```python
from build123d import *

# Parameters (mm, degrees)
SKETCH_1_W                = 130
SKETCH_1_H                = 15
EXTRUDE_1_DEPTH           = 8
CUT_EXTRUDE_10_REACH      = 133.107
SKETCH_17_R               = 3
CUT_EXTRUDE_12_REACH      = 133.107
SKETCH_15_R               = 3
SKETCH_22_W               = 8
SKETCH_22_H               = 8
EXTRUDE_7_DEPTH           = 5
CUT_EXTRUDE_18_DEPTH      = 1.5
SKETCH_25_W               = 4.62
SKETCH_25_H               = 1.5
CUT_EXTRUDE_19_DEPTH      = 4
FILLET_8_R                = 3
FILLET_9_R                = 2
FILLET_10_R               = 2
FILLET_11_R               = 3
CUT_EXTRUDE_20_DEPTH      = 15.5
CUT_EXTRUDE_20_DEPTH_BACK = 28.5
SKETCH_21_R               = 1
FILLET_12_R               = 10
FILLET_13_R               = 5


# Some blends are built 0.0001 mm under size
with BuildPart() as part:
    # 草图1 → 凸台-拉伸1 (new body)
    with BuildSketch(Plane(origin=(0, 0, 0), x_dir=(0, 0, -1), z_dir=(1, 0, 0))):
        with Locations((65, 7.5)):
            Rectangle(SKETCH_1_W, SKETCH_1_H)
    extrude(amount=EXTRUDE_1_DEPTH)

    # 草图17 → 切除-拉伸10 (cut, up to next)
    with BuildSketch(Plane.ZY, mode=Mode.PRIVATE) as cut_extrude_10_sk1:
        with Locations((-115, 7.5)):
            Circle(SKETCH_17_R)
    cut_extrude_10_tool1 = extrude(cut_extrude_10_sk1.sketch, amount=-CUT_EXTRUDE_10_REACH, mode=Mode.PRIVATE) & part.part
    # 草图17 → 切除-拉伸10 (cut, up to next)
    with BuildSketch(Plane.ZY, mode=Mode.PRIVATE) as cut_extrude_10_sk2:
        with Locations((-95, 7.5)):
            Circle(SKETCH_17_R)
    cut_extrude_10_tool2 = extrude(cut_extrude_10_sk2.sketch, amount=-CUT_EXTRUDE_10_REACH, mode=Mode.PRIVATE) & part.part
    # 草图17 → 切除-拉伸10 (cut, up to next)
    with BuildSketch(Plane.ZY, mode=Mode.PRIVATE) as cut_extrude_10_sk3:
        with Locations((-75, 7.5)):
            Circle(SKETCH_17_R)
    cut_extrude_10_tool3 = extrude(cut_extrude_10_sk3.sketch, amount=-CUT_EXTRUDE_10_REACH, mode=Mode.PRIVATE) & part.part
    # 草图17 → 切除-拉伸10 (cut, up to next)
    with BuildSketch(Plane.ZY, mode=Mode.PRIVATE) as cut_extrude_10_sk4:
        with Locations((-55, 7.5)):
            Circle(SKETCH_17_R)
    cut_extrude_10_tool4 = extrude(cut_extrude_10_sk4.sketch, amount=-CUT_EXTRUDE_10_REACH, mode=Mode.PRIVATE) & part.part
    # 草图17 → 切除-拉伸10 (cut, up to next)
    with BuildSketch(Plane.ZY, mode=Mode.PRIVATE) as cut_extrude_10_sk5:
        with Locations((-35, 7.5)):
            Circle(SKETCH_17_R)
    cut_extrude_10_tool5 = extrude(cut_extrude_10_sk5.sketch, amount=-CUT_EXTRUDE_10_REACH, mode=Mode.PRIVATE) & part.part
    add(cut_extrude_10_tool1.solids().sort_by_distance((0, 7.5, -115))[0], mode=Mode.SUBTRACT)
    add(cut_extrude_10_tool2.solids().sort_by_distance((0, 7.5, -95))[0], mode=Mode.SUBTRACT)
    add(cut_extrude_10_tool3.solids().sort_by_distance((0, 7.5, -75))[0], mode=Mode.SUBTRACT)
    add(cut_extrude_10_tool4.solids().sort_by_distance((0, 7.5, -55))[0], mode=Mode.SUBTRACT)
    add(cut_extrude_10_tool5.solids().sort_by_distance((0, 7.5, -35))[0], mode=Mode.SUBTRACT)

    # 草图15 → 切除-拉伸12 (cut, up to next)
    with BuildSketch(Plane.ZY, mode=Mode.PRIVATE) as cut_extrude_12_sk1:
        with Locations((-6.4, 7.5)):
            Circle(SKETCH_15_R)
    cut_extrude_12_tool1 = extrude(cut_extrude_12_sk1.sketch, amount=-CUT_EXTRUDE_12_REACH, mode=Mode.PRIVATE) & part.part
    add(cut_extrude_12_tool1.solids().sort_by_distance((0, 7.5, -6.4))[0], mode=Mode.SUBTRACT)

    # 草图22 → 凸台-拉伸7 (add)
    with BuildSketch(Plane(origin=(0, 15, 0), x_dir=(1, 0, 0), z_dir=(0, 1, 0))):
        with Locations((4, 6.4)):
            Rectangle(SKETCH_22_W, SKETCH_22_H)
    extrude_7 = extrude(amount=EXTRUDE_7_DEPTH)

    # 草图24 → 切除-拉伸18 (cut)
    with BuildSketch(Plane(origin=(0, 15, 0), x_dir=(1, 0, 0), z_dir=(0, 1, 0))):
        Polygon((4, 4.090598923), (6, 5.245299462), (6, 7.554700538), (4, 8.709401077), (2, 7.554700538), (2, 5.245299462), align=None)
    cut_extrude_18 = extrude(amount=CUT_EXTRUDE_18_DEPTH, mode=Mode.SUBTRACT)

    # 草图25 → 切除-拉伸19 (cut)
    with BuildSketch(Plane(origin=(8, 0, 0), x_dir=(0, 0, -1), z_dir=(1, 0, 0))):
        with Locations((6.4, 15.75)):
            Rectangle(SKETCH_25_W, SKETCH_25_H)
    cut_extrude_19 = extrude(amount=-CUT_EXTRUDE_19_DEPTH, mode=Mode.SUBTRACT)

    # 圆角8
    # the kernel refuses this fillet: 3 mm, written as the material it adds along each edge
    with BuildSketch(Plane(origin=(8, 15, -2.4), x_dir=(0, 1.5846583304811187e-12, 1.0), z_dir=(-1, 0, 0))) as fillet_8_piece_1:
        with BuildLine():
            CenterArc((3, 2.939387691), FILLET_8_R, 180, 78.463040967)
            Line((0, 2.939387691), (-0.06, 2.939387691))
            Line((-0.06, 2.939387691), (-0.06, 0))
            Line((-0.06, 0), (0, -0.06))
            ThreePointArc((0, -0.06), (1.2, -0.06), (2.388, -0.058787754))
            Line((2.388, -0.058787754), (2.4, 0))
        make_face()
    extrude(amount=8)
    with BuildSketch(Plane(origin=(0, 15, -10.4), x_dir=(0, 0, -1), z_dir=(1, 0, 0))) as fillet_8_piece_2:
        with BuildLine():
            CenterArc((FILLET_8_R, FILLET_8_R), FILLET_8_R, 180, 90)
            Line((0, FILLET_8_R), (-FILLET_8_R * 0.02, FILLET_8_R))
            Line((-FILLET_8_R * 0.02, FILLET_8_R), (-FILLET_8_R * 0.02, -FILLET_8_R * 0.02))
            Line((-FILLET_8_R * 0.02, -FILLET_8_R * 0.02), (FILLET_8_R, -FILLET_8_R * 0.02))
            Line((FILLET_8_R, -FILLET_8_R * 0.02), (FILLET_8_R, 0))
        make_face()
    extrude(amount=8)

    # 圆角9
    fillet_9_edges = [part.edges().sort_by_distance(p)[0] for p in [
        (4, 20, -2.4),
        (4, 20, -10.4),
    ]]
    fillet(fillet_9_edges, radius=FILLET_9_R - 0.0001)  # a hair under: the kernel refuses the full size

    # 镜向6: 凸台-拉伸7, 切除-拉伸18, 切除-拉伸19 across plane
    add(extrude_7.mirror(Plane.ZX.offset(7.5)))
    add(cut_extrude_18.mirror(Plane.ZX.offset(7.5)), mode=Mode.SUBTRACT)
    add(cut_extrude_19.mirror(Plane.ZX.offset(7.5)), mode=Mode.SUBTRACT)

    # 圆角10
    fillet_10_edges = [part.edges().sort_by_distance(p)[0] for p in [
        (4, -5, -10.4),
        (4, -5, -2.4),
    ]]
    fillet(fillet_10_edges, radius=FILLET_10_R)

    # 圆角11
    # the kernel refuses this fillet: 3 mm, written as the material it adds along each edge
    with BuildSketch(Plane(origin=(8, 0, -2.4), x_dir=(0, -1, 0), z_dir=(-1, 0, 0))) as fillet_11_piece_1:
        with BuildLine():
            CenterArc((2.939387691, 3), FILLET_11_R, 191.536959033, 78.463040967)
            Line((0, 2.4), (-0.058787754, 2.388))
            ThreePointArc((-0.058787754, 2.388), (-0.06, 1.2), (-0.06, 0))
            Line((-0.06, 0), (0, -0.06))
            Line((0, -0.06), (2.939387691, -0.06))
            Line((2.939387691, -0.06), (2.939387691, 0))
        make_face()
    extrude(amount=8)
    with BuildSketch(Plane(origin=(0, 0, -10.4), x_dir=(0, -1, 0), z_dir=(1, 0, 0))) as fillet_11_piece_2:
        with BuildLine():
            CenterArc((FILLET_11_R, FILLET_11_R), FILLET_11_R, 180, 90)
            Line((0, FILLET_11_R), (-FILLET_11_R * 0.02, FILLET_11_R))
            Line((-FILLET_11_R * 0.02, FILLET_11_R), (-FILLET_11_R * 0.02, -FILLET_11_R * 0.02))
            Line((-FILLET_11_R * 0.02, -FILLET_11_R * 0.02), (FILLET_11_R, -FILLET_11_R * 0.02))
            Line((FILLET_11_R, -FILLET_11_R * 0.02), (FILLET_11_R, 0))
        make_face()
    extrude(amount=8)

    # 草图21 → 切除-拉伸20 (cut, two sides: drawn at the far end of the back side and taken through both)
    with BuildSketch(Plane(origin=(0, 15, 0), x_dir=(1, 0, 0), z_dir=(0, 1, 0)).offset(-CUT_EXTRUDE_20_DEPTH_BACK)):
        with Locations(Location((4, 6.4, 0), (0, 0, 90))):
            Circle(SKETCH_21_R)
    extrude(amount=CUT_EXTRUDE_20_DEPTH + CUT_EXTRUDE_20_DEPTH_BACK, mode=Mode.SUBTRACT)

    # 圆角12
    fillet_12_edges = [part.edges().sort_by_distance(p)[0] for p in [
        (4, 15, 0),
        (4, 0, 0),
    ]]
    fillet(fillet_12_edges, radius=FILLET_12_R)

    # 圆角13
    fillet_13_edges = [part.edges().sort_by_distance(p)[0] for p in [
        (4, 15, -130),
        (4, 0, -130),
    ]]
    fillet(fillet_13_edges, radius=FILLET_13_R)


solid = part.part
```
Design review of the part built by this model. Coordinates are the model's own, in mm. A direction names the side the tool comes from. Round coordinates to 2 decimals unless told otherwise and drop trailing zeros. Order: outer loops, then holes, each group sorted by start corner. A loop starts at its lowest first (then second) coordinate and runs counter-clockwise, first axis right, second up. Notation, with made-up numbers: (-33, -24) - (-21, -24) arc R23 ccw to (-21, -2) - close; hole circle Ø2 at (-24.5, 83.5). An arc over 180 degrees is marked (long way). One line per question, with ' | ' between items.
Item 1: Machinability: for faces 1 (the face through (6, -1.5, -6)), 2 (the face through (4, 15, -68)), 3 (the face through (4.06, 19.43, -3)), which of the approach directions +Z, -Z, +X, -X, +Y, -Y give a long, thin tool a straight path to every point of the face, cutting with its end or side? Answer none if there is none.
Checks:
face 1: +X | face 2: -Z, +X, -X, +Y | face 3: +Z, +X, -X, +Y
Item 2: Take a section at A-A, the plane z = -75. Write out the cut boundary in (x, y).
Checks:
outline: (0, 0) - (8, 0) - (8, 4.5) - (0, 4.5) - close; (0, 10.5) - (8, 10.5) - (8, 15) - (0, 15) - close
Item 3: Draft analysis for pull direction X (two halves, no side actions). For faces 4 (the face through (3.7, 12.631, -7.354)), 5 (the face through (3.94, -0.86, -11.3)), state which applies: +X half, -X half, draft (parallel to the pull), parting line (faces both ways), or undercut.
Checks:
face 4: undercut | face 5: draft
Item 4: Wall thickness on line 1 (Y direction, x = 2.5, z = -55); line 2 (Z direction, x = 1.5, y = 18); line 3 (Y direction, x = 6.75, z = -34): over which ranges is each line inside the solid? List them lowest first. Write a range as [from, to].
Checks:
line 1: [0, 4.5], [10.5, 15] | line 2: [-10.4, -2.4] | line 3: [0, 4.67], [10.33, 15]
Item 5: Take a section at B-B, the plane y = 7.5. Write out the cut boundary in (x, z), then the cut area to 3 significant figures.
Checks:
outline: (0, -130) - (8, -130) - (8, -118) - (0, -118) - close; (0, -112) - (8, -112) - (8, -98) - (0, -98) - close; (0, -92) - (8, -92) - (8, -78) - (0, -78) - close; (0, -72) - (8, -72) - (8, -58) - (0, -58) - close; (0, -52) - (8, -52) - (8, -38) - (0, -38) - close; (0, -32) - (8, -32) - (8, -9.4) - (0, -9.4) - close; (0, -3.4) - (8, -3.4) - (8, 0) - (0, 0) - close | area: 752 mm²
Item 6: For P1, Ø1.2, axis at x = 4, z = -6.4, coming from the -Y side; P2, Ø1.6, axis at x = 6, y = 15.5, coming from the +Z side; P3, Ø2, axis at x = 7, z = -39, coming from the +Y side; P4, Ø2.5, axis at x = 4, z = -70.5, coming from the -Y side, all flat-tipped, find the tip position at first contact; note any pin that passes through.
Checks:
P1: through | P2: z = -0.97 | P3: y = 15 | P4: y = 0
